Verification items for the finished model (mm, model axes). Face numbers are marked on the shaded views. A direction names the side the tool comes from. Round coordinates to 2 decimals unless told otherwise and drop trailing zeros. Write each loop counter-clockwise with the first axis right and the second up, starting at its lowest first coordinate (ties: lowest second). Pieces come first, ordered by that corner, then holes. Notation, with made-up numbers: M -29,16 L 7,16 A21 cw 7,37 Z; hole C 64,63 d8. An arc over 180 degrees is marked long. One line per item, written item: value. Start each with the question number.
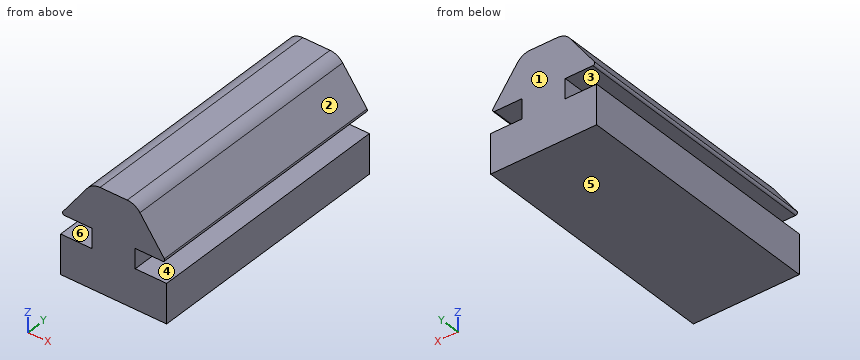
from build123d import *

# Parameters (mm, degrees)
F0_W     = 2.75
F0_H     = 5.5
F1_DEPTH = 32.5
F2_R     = 2
F3_R     = 0.25


with BuildPart() as f1:
    # F0 (on Front) → F1 (new body)
    with BuildSketch(Plane.XZ):
        with Locations((1.375, 2.75)):
            Rectangle(F0_W, F0_H)
        Polygon((0, 0), (-2.75, 0), (-2.75, -2.5), (-6.75, -2.5), (-6.75, -7.5), (6.75, -7.5), (6.75, -2.5), (2.75, -2.5), (2.75, 0), align=None)
        Polygon((2.75, 5.5), (2.75, 0), (6.75, 0), align=None)
        with Locations((-1.375, 2.75)):
            Rectangle(F0_W, F0_H)
        Polygon((-2.75, 5.5), (-6.75, 0), (-2.75, 0), align=None)
    extrude(amount=F1_DEPTH)

    # F2
    f2_edges = [f1.edges().sort_by_distance(p)[0] for p in [
        (2.75, -16.25, 5.5),
        (-2.75, -16.25, 5.5),
    ]]
    fillet(f2_edges, radius=F2_R)

    # F3
    f3_edges = [f1.edges().sort_by_distance(p)[0] for p in [
        (6.75, -16.25, 0),
        (-6.75, -16.25, 0),
    ]]
    fillet(f3_edges, radius=F3_R)


solid = f1.part
1) Cross-section at C-C (z = -2). Record the boundary of the cut face in (x, y).
2) Mould release check, pull along Z, two halves, no side actions. Record for the marked faces 1, 2 and 3: pulls with the +Z half, pulls with the -Z half, needs draft (parallel to the pull), parting line crosses it, or undercut.
3) Cross-section at B-B (x = 3.75). Record the boundary of the cut face in (y, z) (3 decimals), then the cut area to 3 significant figures.
4) Access from +Z, -Z, +X, -X, +Y, -Y to the whole of each face (thin tool, end or side, straight path). Record for the marked faces 4, 5 and 6.
5) Thickness scan on line 1 (X direction, y = -9, z = -1); line 2 (Z direction, x = -3.5, y = -11); line 3 (Z direction, x = 4.25, y = -3). Record the ranges inside material, lowest first.
6) Gauge pin test, flat ends, axial feed: pin 1 Ø2 at (x, y) = (5, -15) entering from +Z; pin 2 Ø5 at (x, z) = (0, 0) entering from +Y; pin 3 Ø0.8 at (y, z) = (-10.5, -1) entering from +X; pin 4 Ø1 at (y, z) = (-15, 3.5) entering from -X. Record the tip position at first contact, or that the pin passes through.
7) Cross-section at A-A (y = -17.5). Record the boundary of the cut face in (x, z), then the cut area to 3 significant figures.
Results below:
1. outline: M -2.75,-32.5 L 2.75,-32.5 L 2.75,0 L -2.75,0 Z
2. face 1: needs draft
2. face 2: pulls with the +Z half
2. face 3: undercut
3. outline: M -32.5,-7.5 L 0,-7.5 L 0,-2.5 L -32.5,-2.5 Z; M -32.5,0 L 0,0 L 0,4.125 L -32.5,4.125 Z
3. area: 297 mm²
4. face 4: +X, +Y, -Y
4. face 5: -Z, +X, -X, +Y, -Y
4. face 6: -X, +Y, -Y
5. line 1: x = -2.75 to 2.75
5. line 2: z = -7.5 to -2.5, 0 to 4.47
5. line 3: z = -7.5 to -2.5, 0 to 3.44
6. pin 1: stops at z = 3.78
6. pin 2: stops at y = 0
6. pin 3: stops at x = 2.75
6. pin 4: stops at x = -4.57
7. outline: M -6.75,-7.5 L 6.75,-7.5 L 6.75,-2.5 L 2.75,-2.5 L 2.75,0 L 6.26,0 A0.25 ccw 6.46,0.4 L 3.35,4.68 A2 ccw 1.73,5.5 L -1.73,5.5 A2 ccw -3.35,4.68 L -6.46,0.4 A0.25 ccw -6.26,0 L -2.75,0 L -2.75,-2.5 L -6.75,-2.5 Z
7. area: 133 mm²
